Work out the finished part from the listing and answer in its coordinate system (mm). A direction names the side the tool comes from. Coordinates: 2 decimals unless noted, no trailing zeros. Order: outer loops, then holes, each group sorted by start corner. A loop starts at its lowest first (then second) coordinate and runs counter-clockwise, first axis right, second up.
```python
from build123d import *

# Parameters (mm, degrees)
F1_DEPTH = 15
F2_W     = 18.92
F2_H     = 9.92
F3_DEPTH = 6.35


with BuildPart() as f1:
    # F0 (on Top) → F1 (new body)
    with BuildSketch(Plane.XY):
        Polygon((-25, 12), (-25, 0), (-25, -12), (25, -12), (25, 0), (25, 12), align=None)
    extrude(amount=F1_DEPTH)

    # F2 (on face) → F3 (cut)
    with BuildSketch(Plane.YZ.offset(25)):
        with Locations((0, 7.5)):
            Rectangle(F2_W, F2_H)
    extrude(amount=-F3_DEPTH, mode=Mode.SUBTRACT)


solid = f1.part
```
1. For faces 4 (the flat face through (22, 0, 2.54)), 5 (the flat face through (0, 12, 7)), determine the directions among +Z, -Z, +X, -X, +Y, -Y from which every point of the face is accessible in a straight line to the end or side of a thin tool.
2. Consider probe 1 along Y at (x, z) = (21, 4.25); probe 2 along X at (y, z) = (-6.75, 5.5). Determine where each line is inside the solid, lowest interval first.
3. The part is cut by section A-A (z = 6.5). Determine the outline of the cut face in (x, y), plus the area to 3 significant figures.
4. The part is cut by section B-B (y = -3.75). Determine the outline of the cut face in (x, z).
5. A flat-ended cylindrical pin translates along its axis: pin 1 (3 mm diameter, centred on y = 2.5, z = 7, fed in from +X). Find the tip coordinate at first contact, or state that the pin passes through.
6. The mould has two halves that part along Z. Classify faces 1 (the flat face through (22, -9.46, 7)), 2 (the flat face through (0, -12, 7)), 3 (the flat face through (0, 0, 0)): released by +Z, released by -Z, zero draft, split by the parting line, or undercut.
7. The part is cut by section C-C (x = 21.5). Determine the outline of the cut face in (y, z), plus the area to 3 significant figures.
Worked out:
1. face 4: +X
1. face 5: +Z, -Z, +X, -X, +Y
2. probe 1: y = -12 to -9.46, 9.46 to 12
2. probe 2: x = -25 to 18.65
3. outline: (-25, -12) - (25, -12) - (25, -9.46) - (18.65, -9.46) - (18.65, 9.46) - (25, 9.46) - (25, 12) - (-25, 12) - close
3. area: 1,080 mm2
4. outline: (-25, 0) - (25, 0) - (25, 2.54) - (18.65, 2.54) - (18.65, 12.46) - (25, 12.46) - (25, 15) - (-25, 15) - close
5. pin 1: stops at x = 18.65
6. face 1: undercut
6. face 2: zero draft
6. face 3: released by -Z
7. outline: (-12, 0) - (12, 0) - (12, 15) - (-12, 15) - close; hole (-9.46, 2.54) - (9.46, 2.54) - (9.46, 12.46) - (-9.46, 12.46) - close
7. area: 172 mm2
